```python
from build123d import *

# Parameters (mm, degrees)
SKETCH1_R           = 5
BOSS_EXTRUDE1_DEPTH = 5


with BuildPart() as part:
    # Sketch1 → Boss-Extrude1 (new body)
    with BuildSketch(Plane.XY):
        with BuildLine():
            Line((-15.492752905, 12.648106871), (-15.492752905, -12.648106871))
            ThreePointArc((-15.492752905, -12.648106871), (0, -20), (15.492752905, -12.648106871))
            Line((15.492752905, -12.648106871), (15.492752905, 12.648106871))
            ThreePointArc((15.492752905, 12.648106871), (0, 20), (-15.492752905, 12.648106871))
        make_face()
        Circle(SKETCH1_R, mode=Mode.SUBTRACT)
    extrude(amount=BOSS_EXTRUDE1_DEPTH)


solid = part.part
```
Check sheet for the modelled part. Datum: model origin and axes. Units: mm. Coordinates: 2 decimals unless noted, no trailing zeros. Loops run counter-clockwise (first coordinate to the right, second up) from the corner with the lowest first, then second, coordinate; pieces in that order, holes last.
1) Sectioned sample at B-B (x = 0). Record the boundary of the cut face in (y, z), and give its area (3 significant figures).
2) Release check for a two-part mould opening along Y. For faces 1 (the face through (-1.08, -4.88, 2.46)), 2 (the face through (-4, 5, 0)), 3 (the face through (0, -20, 2)), 4 (the face through (0, 20, 2)) record: released by +Y, released by -Y, zero draft, split by the parting line, or undercut.
3) Sectioned sample at C-C (z = 2.55). Record the boundary of the cut face in (x, y), and give its area (3 significant figures).
4) Material ranges on probe 1 along Y at (x, z) = (1, 0.75); probe 2 along Y at (x, z) = (-1.5, 1.15); probe 3 along X at (y, z) = (-17.5, 2.4), recorded low to high.
5) Sectioned sample at D-D (y = -17.5). Record the boundary of the cut face in (x, z), and give its area (3 significant figures).
6) Gauge pin test, flat ends, axial feed: pin 1 (3 mm diameter, centred on x = 2, z = 3.5, fed in from -Y); pin 2 (5 mm diameter, centred on x = -6, y = 15.5, fed in from -Z). Record the tip position at first contact, or that the pin passes through.
7) Sectioned sample at A-A (y = -3). Record the boundary of the cut face in (x, z).
Check sheet entries:
1. outline: (-20, 0) - (-5, 0) - (-5, 5) - (-20, 5) - close; (5, 0) - (20, 0) - (20, 5) - (5, 5) - close
1. area: 150 mm2
2. face 1: undercut
2. face 2: zero draft
2. face 3: released by -Y
2. face 4: released by +Y
3. outline: (-15.49, -12.65) arc R20 ccw to (15.49, -12.65) - (15.49, 12.65) arc R20 ccw to (-15.49, 12.65) - close; hole circle Ø10 at (0, 0)
3. area: 1,020 mm2
4. probe 1: y = -19.97 to -4.9, 4.9 to 19.97
4. probe 2: y = -19.94 to -4.77, 4.77 to 19.94
4. probe 3: x = -9.68 to 9.68
5. outline: (-9.68, 0) - (9.68, 0) - (9.68, 5) - (-9.68, 5) - close
5. area: 96.8 mm2
6. pin 1: stops at y = -19.99
6. pin 2: stops at z = 0
7. outline: (-15.49, 0) - (-4, 0) - (-4, 5) - (-15.49, 5) - close; (4, 0) - (15.49, 0) - (15.49, 5) - (4, 5) - close
